Part model, mm, in its own coordinate system. A direction names the side the tool comes from. Give positions to 0.01 mm unless a question says otherwise; leave off trailing zeros. Write each loop counter-clockwise with the first axis right and the second up, starting at its lowest first coordinate (ties: lowest second). Pieces come first, ordered by that corner, then holes. Notation, with made-up numbers: M 78,-16.5 L 106,-16.5 A11 ccw 106,3.5 Z; hole C 51.25,76 d9. An arc over 180 degrees is marked long. Use a Markdown table: item, result.
```python
from build123d import *

# Parameters (mm, degrees)
SKETCH_1_R          = 5
EXTRUDE_1_DEPTH     = 7
SKETCH_2_R          = 2.55
CUT_EXTRUDE_1_DEPTH = 31.374989712
CUT_EXTRUDE_2_DEPTH = 40.570696228
FILLET_2_R          = 1
SKETCH_5_R          = 4.95
EXTRUDE_2_DEPTH     = 3


with BuildPart() as part:
    # 草图1 → 凸台-拉伸1 (new, symmetric)
    with BuildSketch(Plane.XY):
        Polygon((-21, 0), (21, 0), (21, 12), (9, 12), (9, 32.8), (-9, 32.8), (-9, 12), (-21, 12), align=None)
        with Locations((0, 20)):
            Circle(SKETCH_1_R, mode=Mode.SUBTRACT)
    extrude(amount=EXTRUDE_1_DEPTH, both=True)

    # 草图2 → 切除-拉伸1 (cut, through all)
    with BuildSketch(Plane(origin=(0, 12, 0), x_dir=(1, 0, 0), z_dir=(0, 1, 0))):
        with Locations(Location((16, 0, 0), (0, 0, 270))):
            Circle(SKETCH_2_R)
        with Locations(Location((-16, 0, 0), (0, 0, 90))):
            Circle(SKETCH_2_R)
    extrude(amount=-CUT_EXTRUDE_1_DEPTH, mode=Mode.SUBTRACT)

    # 草图4 → 切除-拉伸2 (cut, through all)
    with BuildSketch(Plane(origin=(0, 32.8, 0), x_dir=(1, 0, 0), z_dir=(0, 1, 0))):
        Polygon((-9, 3), (-3, 3), (-3, -3), (-9, -3), (-9, -7), (-21, -7), (-21, 7), (-9, 7), align=None)
    extrude(amount=-CUT_EXTRUDE_2_DEPTH, mode=Mode.SUBTRACT)

    # 圆角2
    fillet_2_edges = [part.edges().sort_by_distance(p)[0] for p in [
        (9, 12, 0),
    ]]
    fillet(fillet_2_edges, radius=FILLET_2_R)

    # 草图5 → 凸台-拉伸2 (add)
    with BuildSketch(Plane.XZ):
        with Locations(Location((5, 0, 0), (0, 0, 180))):
            Circle(SKETCH_5_R)
    extrude(amount=EXTRUDE_2_DEPTH)


solid = part.part
```
1. Drill centre lines: L1, parallel to X at y = 5, z = 0; L2, parallel to Y at x = 0, z = 1; L3, parallel to Z at x = -6, y = 4. Where is each one in solid material? Low to high.
Findings below:
| item | result |
|---|---|
| L1 | -3 to 13.45, 18.55 to 21 |
| L2 | 0 to 15, 25 to 32.8 |
| L3 | -7 to -3, 3 to 7 |
2. Cut at D-D, the plane z = 6. Give the cut face in (x, y).
Findings below:
| item | result |
|---|---|
| outline | M -9,0 L 21,0 L 21,12 L 10,12 A1 cw 9,13 L 9,32.8 L -9,32.8 Z; hole C 0,20 d10 |
3. Cut at A-A, the plane x = 16. Give the cut face in (y, z), then the cut area to 3 significant figures.
Findings below:
| item | result |
|---|---|
| outline | M 0,-7 L 12,-7 L 12,-2.55 L 0,-2.55 Z; M 0,2.55 L 12,2.55 L 12,7 L 0,7 Z |
| area | 107 mm2 |
4. Cut at C-C, the plane y = 20. Give the cut face in (x, z), then the cut area to 3 significant figures.
Findings below:
| item | result |
|---|---|
| outline | M -9,-7 L -5,-7 L -5,-3 L -9,-3 Z; M -9,3 L -5,3 L -5,7 L -9,7 Z; M 5,-7 L 9,-7 L 9,7 L 5,7 Z |
| area | 88.0 mm2 |
5. Drop flat-ended pins along their axis: P1, Ø4, axis at x = 14, z = 3, coming from the +Y side; P2, Ø4.5, axis at x = 16, z = 0, coming from the +Y side; P3, Ø1.8, axis at y = 29.5, z = 0, coming from the -X side. Give the stop position or say it passes through.
Findings below:
| item | result |
|---|---|
| P1 | y = 12 |
| P2 | through |
| P3 | x = -3 |
6. Cut at B-B, the plane z = 0. Give the cut face in (x, y), then the cut area to 3 significant figures.
Findings below:
| item | result |
|---|---|
| outline | M -3,0 L 0.05,0 L 0.05,-3 L 9.95,-3 L 9.95,0 L 13.45,0 L 13.45,12 L 10,12 A1 cw 9,13 L 9,32.8 L -3,32.8 L -3,24 A5 cw long -3,16 Z; M 18.55,0 L 21,0 L 21,12 L 18.55,12 Z |
| area | 439 mm2 |
7. Tool access for faces 1 (the flat face through (9, 23, 0)), 2 (the flat face through (-6, 17, -3)), 3 (the flat face through (-9, 17, -5)): list every direction of +Z, -Z, +X, -X, +Y, -Y with a clear straight run to the whole face (end or side of a thin tool).
Findings below:
| item | result |
|---|---|
| face 1 | +Z, -Z, +X, +Y |
| face 2 | -X, +Y, -Y |
| face 3 | +Z, -Z, -X, +Y, -Y |
8. Two-plate mould, pull along X, no slides. Class faces 4 (the cylindrical face through (4.619, 18.085, -0.098)), 5 (the cylindrical face through (13.51, 6.08, -0.55)), 6 (the flat face through (5, -3, 0)), 7 (the cylindrical face through (0.28, -1.48, -1.49)): released by +X, released by -X, zero draft, split by the parting line, or undercut.
Findings below:
| item | result |
|---|---|
| face 4 | undercut |
| face 5 | undercut |
| face 6 | zero draft |
| face 7 | split by the parting line |
